```python
from build123d import *

# Parameters (mm, degrees)
BOSS_EXTRUDE1_DEPTH     = 2.413
CHAMFER1_SIZE           = 19.05
CHAMFER2_SIZE           = 5.08
CUT_EXTRUDE1_DEPTH      = 108.790085671
CUT_EXTRUDE1_DEPTH_BACK = 108.790085671
SKETCH2_R               = 2.54


with BuildPart() as part:
    # Sketch1 → Boss-Extrude1 (new body)
    with BuildSketch(Plane(origin=(0, 0, 0), x_dir=(1, 0, 0), z_dir=(0, 1, 0))):
        Polygon((25.4, 76.2), (25.4, 25.4), (76.2, 25.4), (76.2, 0), (0, 0), (0, 76.2), align=None)
    extrude(amount=BOSS_EXTRUDE1_DEPTH)

    # Chamfer1
    chamfer1_edges = [part.edges().sort_by_distance(p)[0] for p in [
        (25.4, 1.2065, -25.4),
    ]]
    chamfer(chamfer1_edges, length=CHAMFER1_SIZE)

    # Chamfer2
    chamfer2_edges = [part.edges().sort_by_distance(p)[0] for p in [
        (0, 1.2065, -76.2),
        (25.4, 1.2065, -76.2),
        (76.2, 1.2065, -25.4),
        (76.2, 1.2065, 0),
        (0, 1.2065, 0),
    ]]
    chamfer(chamfer2_edges, length=CHAMFER2_SIZE)

    # Sketch2 → Cut-Extrude1 (cut, two sides: drawn at the far end of the back side and taken through both)
    with BuildSketch(Plane(origin=(0, 0, 0), x_dir=(1, 0, 0), z_dir=(0, 1, 0)).offset(-CUT_EXTRUDE1_DEPTH_BACK)):
        with Locations(Location((12.7, 12.7, 0), (0, 0, 270))):
            Circle(SKETCH2_R)
        with Locations(Location((12.7, 38.1, 0), (0, 0, 270))):
            Circle(SKETCH2_R)
        with Locations(Location((38.1, 12.7, 0), (0, 0, 270))):
            Circle(SKETCH2_R)
        with Locations(Location((12.7, 63.5, 0), (0, 0, 270))):
            Circle(SKETCH2_R)
        with Locations(Location((63.5, 12.7, 0), (0, 0, 270))):
            Circle(SKETCH2_R)
    extrude(amount=CUT_EXTRUDE1_DEPTH + CUT_EXTRUDE1_DEPTH_BACK, mode=Mode.SUBTRACT)


solid = part.part
```
Build history of the part. All positions in model axes, mm. A direction names the side the tool comes from. Give positions to 0.01 mm unless a question says otherwise; leave off trailing zeros. Loops run counter-clockwise (first coordinate to the right, second up) from the corner with the lowest first, then second, coordinate; pieces in that order, holes last.
Item 1: Pull direction X, two halves, no side cores. Call faces 3 (the face through (39, 1, 0)), 4 (the face through (73.7, 1.19, -22.82)), 5 (the face through (15.22, 1.19, -38.43)): released by +X, released by -X, zero draft, split by the parting line, or undercut.
Answers follow:
face 3: zero draft
face 4: released by +X
face 5: undercut
Item 2: Flat gauge pins, fed straight in: pin 1 (6 mm diameter, centred on x = 12.7, z = -12.7, fed in from +Y); pin 2 (0.7 mm diameter, centred on y = 1.5, z = -59.5, fed in from +X); pin 3 (0.7 mm diameter, centred on x = 57.5, y = 1, fed in from -Z). Where does each tip first touch, or does it go through?
Answers follow:
pin 1: stops at y = 2.41
pin 2: stops at x = 25.4
pin 3: stops at z = -25.4
Item 3: Slice it at C-C, the plane x = 63.5. List the corners of the cut face in (y, z), and give its area (3 significant figures).
Answers follow:
outline: (0, -25.4) - (2.41, -25.4) - (2.41, -15.24) - (0, -15.24) - close; (0, -10.16) - (2.41, -10.16) - (2.41, 0) - (0, 0) - close
area: 49.0 mm2
Item 4: Slice it at B-B, the plane z = -12.7. List the corners of the cut face in (x, y), and give its area (3 significant figures).
Answers follow:
outline: (0, 0) - (10.16, 0) - (10.16, 2.41) - (0, 2.41) - close; (15.24, 0) - (35.56, 0) - (35.56, 2.41) - (15.24, 2.41) - close; (40.64, 0) - (60.96, 0) - (60.96, 2.41) - (40.64, 2.41) - close; (66.04, 0) - (76.2, 0) - (76.2, 2.41) - (66.04, 2.41) - close
area: 147 mm2
Item 5: Drill centre lines: line 1 (Z direction, x = 12.7, y = 0.95); line 2 (X direction, y = 1.9, z = -12.7); line 3 (Z direction, x = 63.5, y = 1.85). Where is each one in solid material? Low to high.
Answers follow:
line 1: z = -76.2 to -66.04, -60.96 to -40.64, -35.56 to -15.24, -10.16 to 0
line 2: x = 0 to 10.16, 15.24 to 35.56, 40.64 to 60.96, 66.04 to 76.2
line 3: z = -25.4 to -15.24, -10.16 to 0
Item 6: Slice it at D-D, the plane y = 1.55. List the corners of the cut face in (x, z).
Answers follow:
outline: (0, -71.12) - (5.08, -76.2) - (20.32, -76.2) - (25.4, -71.12) - (25.4, -44.45) - (44.45, -25.4) - (71.12, -25.4) - (76.2, -20.32) - (76.2, -5.08) - (71.12, 0) - (5.08, 0) - (0, -5.08) - close; hole circle Ø5.08 at (12.7, -63.5); hole circle Ø5.08 at (12.7, -38.1); hole circle Ø5.08 at (12.7, -12.7); hole circle Ø5.08 at (38.1, -12.7); hole circle Ø5.08 at (63.5, -12.7)
Item 7: Which spindle directions (+Z, -Z, +X, -X, +Y, -Y) get a long thin tool onto all of the face, cutting with end or side? Do faces 1 (the face through (58, 1, -25.4)), 2 (the face through (13, 1, -76.2)). Say none if no direction does.
Answers follow:
face 1: -Z, +X, +Y, -Y
face 2: -Z, +X, -X, +Y, -Y
Item 8: Slice it at A-A, the plane x = 12.7. List the corners of the cut face in (y, z), and give its area (3 significant figures).
Answers follow:
outline: (0, -76.2) - (2.41, -76.2) - (2.41, -66.04) - (0, -66.04) - close; (0, -60.96) - (2.41, -60.96) - (2.41, -40.64) - (0, -40.64) - close; (0, -35.56) - (2.41, -35.56) - (2.41, -15.24) - (0, -15.24) - close; (0, -10.16) - (2.41, -10.16) - (2.41, 0) - (0, 0) - close
area: 147 mm2
